```python
from build123d import *

# Parameters (mm, degrees)
BOSS_EXTRUDE1_DEPTH = 6.35
SKETCH2_W           = 2.54
SKETCH2_H           = 2.54
BOSS_EXTRUDE2_DEPTH = 2.54


with BuildPart() as part:
    # Sketch1 → Boss-Extrude1 (new body)
    with BuildSketch(Plane.XY):
        Polygon((6.35, -3.429), (-6.35, -3.429), (-6.35, 3.429), (-2.54, 3.429), (-2.54, -2.159), (2.54, -2.159), (2.54, 3.429), (6.35, 3.429), align=None)
    extrude(amount=BOSS_EXTRUDE1_DEPTH)

    # Sketch2 → Boss-Extrude2 (add)
    with BuildSketch(Plane.XZ.offset(3.429)):
        with Locations((0, 3.175)):
            Rectangle(SKETCH2_W, SKETCH2_H)
    extrude(amount=BOSS_EXTRUDE2_DEPTH)


solid = part.part
```
The listing builds one solid part. Answer for the finished solid, in the listing's coordinates (mm). A direction names the side the tool comes from. Round coordinates to 2 decimals unless told otherwise and drop trailing zeros. Order: outer loops, then holes, each group sorted by start corner. A loop starts at its lowest first (then second) coordinate and runs counter-clockwise, first axis right, second up. Notation, with made-up numbers: (0.5, -12.5) -> (58.5, -12.5) arc R15 cw to (58.5, -0.5) -> close; hole circle Ø2 at (-37, -25.5). An arc over 180 degrees is marked (long way). Answer as CSV lines item,"result". Start each with the question number.
(1) The part is cut by section D-D (y = -4.5). Determine the outline of the cut face in (x, z) (3 decimals), then the cut area to 3 significant figures.
(2) Find the intervals of material crossed by probe 1 along X at (y, z) = (1.75, 3.5); probe 2 along Y at (x, z) = (5.75, 3.25); probe 3 along Y at (x, z) = (0, 5.5), in increasing order. Write a range as from..to.
(3) Flat-ended cylindrical pins translate along their axes: pin 1 Ø3 at (y, z) = (-4.5, 4) entering from -X; pin 2 Ø2 at (x, z) = (4.5, 2.5) entering from -Y; pin 3 Ø1.3 at (y, z) = (-5, 3) entering from +X; pin 4 Ø0.8 at (x, y) = (0.5, -5.5) entering from +Z (3 decimals). Find the tip coordinate at first contact, or state that the pin passes through.
(4) The part is cut by section A-A (y = 1). Determine the outline of the cut face in (x, z), then the cut area to 3 significant figures.
(5) A tool of negligible diameter and unlimited length cuts with its end or side. For faces 5 (the face through (1.27, -5, 3)), 6 (the face through (0, -5, 4.445)), 7 (the face through (-2.54, 1, 3)), from which of +Z, -Z, +X, -X, +Y, -Y can it reach the whole face along a straight path? Write none if from no direction.
(6) For a pull along X with two mould halves and no side action, classify faces 1 (the face through (0, -3, 0)), 2 (the face through (6.35, 0, 3)), 3 (the face through (-1.27, -5, 3)), 4 (the face through (0, -2.159, 3)) as +X half, -X half, draft (parallel to the pull), parting line (faces both ways), or undercut.
(7) The part is cut by section C-C (x = 1). Determine the outline of the cut face in (y, z) (3 decimals).
(8) The part is cut by section B-B (z = 3). Determine the outline of the cut face in (x, y).
Evaluation:
1,outline,"(-1.27, 1.905) -> (1.27, 1.905) -> (1.27, 4.445) -> (-1.27, 4.445) -> close"
1,area,"6.45 mm²"
2,probe 1,"-6.35..-2.54, 2.54..6.35"
2,probe 2,"-3.43..3.43"
2,probe 3,"-3.43..-2.16"
3,pin 1,"x = -6.35"
3,pin 2,"y = -3.43"
3,pin 3,"x = 1.27"
3,pin 4,"z = 4.445"
4,outline,"(-6.35, 0) -> (-2.54, 0) -> (-2.54, 6.35) -> (-6.35, 6.35) -> close; (2.54, 0) -> (6.35, 0) -> (6.35, 6.35) -> (2.54, 6.35) -> close"
4,area,"48.4 mm²"
5,face 5,"+Z, -Z, +X, -Y"
5,face 6,"+Z, +X, -X, -Y"
5,face 7,"+Z, -Z, +Y"
6,face 1,"draft"
6,face 2,"+X half"
6,face 3,"-X half"
6,face 4,"undercut"
7,outline,"(-5.969, 1.905) -> (-3.429, 1.905) -> (-3.429, 0) -> (-2.159, 0) -> (-2.159, 6.35) -> (-3.429, 6.35) -> (-3.429, 4.445) -> (-5.969, 4.445) -> close"
8,outline,"(-6.35, -3.43) -> (-1.27, -3.43) -> (-1.27, -5.97) -> (1.27, -5.97) -> (1.27, -3.43) -> (6.35, -3.43) -> (6.35, 3.43) -> (2.54, 3.43) -> (2.54, -2.16) -> (-2.54, -2.16) -> (-2.54, 3.43) -> (-6.35, 3.43) -> close"
